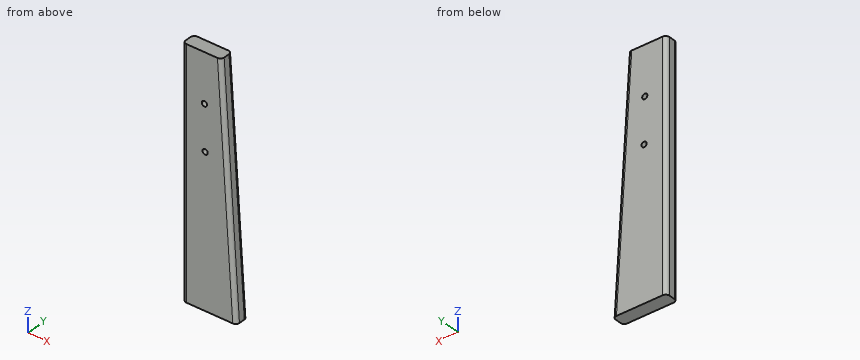
Autodesk Inventor part; units mm, degrees
ref_plane "YZ Plane" through (0, 0, 0) normal (1, 0, 0) x (0, 1, 0)
ref_plane "XZ Plane" through (0, 0, 0) normal (0, 1, 0) x (-1, 0, 0)
ref_plane "XY Plane" through (0, 0, 0) normal (0, 0, 1) x (1, 0, 0)
sketch "Skizze1" plane through (0, 0, 0) normal (0, 1, 0) x (-1, 0, 0)
  line L0 (0, 0) -> (10.3, 0)
  line L1 (10.3, 0) -> (10.3, -65)
  line L2 (10.3, -65) -> (-4.1, -65)
  line L3 (-4.1, -65) -> (0, 0)
  dimension "d0" = 65
  dimension "d1" = 14.4
  dimension "d2" = 10.3
extrude "Extrusion1" add sketch "Skizze1" along normal blind 3.6
sketch "Skizze2" plane through (0, 3.6, 0) normal (0, 1, 0) x (1, 0, 0)
  line L0 (-10.3, 65) -> (-10.3, 0)
  line L1 (-10.3, 0) -> (-10.3, 13)
  line L2 (-10.3, 0) -> (-10.3, 25)
  line L3 (-10.3, 13) -> (-4.5, 13)
  line L4 (-10.3, 25) -> (-4.3, 25)
  point P0 (0, 0)
  dimension "d5" = 13
  dimension "d6" = 25
  dimension "d7" = 5.8
  dimension "d8" = 6
hole "Bohrung1" at (-4.5, 3.6, -13) at (-4.3, 3.6, -25) direction (0, -1, 0) diameter 1.4 end through all
fillet "Rundung1" radius 1 4 edges at (-10.3, 3.6, -32.5) (-10.3, 0, -32.5) (2.05, 3.6, -32.5) (2.05, 0, -32.5)
properties part number "Brillenbuegel"
Source: CAD feature listing. Evaluate the final solid. Frame: model axes, mm. Give positions to 0.01 mm unless a question says otherwise; leave off trailing zeros. Order: outer loops, then holes, each group sorted by start corner. A loop starts at its lowest first (then second) coordinate and runs counter-clockwise, first axis right, second up. Notation, with made-up numbers: (74, 45.25) -> (128, 45.25) arc R30 ccw to (128, 78.25) -> close; hole circle Ø11 at (32, -34.75). An arc over 180 degrees is marked (long way). Write item = value, one per line.
Item 1: Section query A-A (y = 1.7). Output: boundary loops of the cut face in (x, z), then the cut area to 3 significant figures.
Check result:
outline = (-10.3, -65) -> (4.1, -65) -> (0, 0) -> (-10.3, 0) -> close; hole circle Ø1.4 at (-4.5, -13); hole circle Ø1.4 at (-4.3, -25)
area = 800 mm²
Item 2: Contact query for a flat-ended pin moving along its axis: pin 1 (1.5 mm diameter, centred on y = 0.5, z = -27, fed in from +X). Output: stop coordinate, or through.
Check result:
pin_1 = 1.74
Item 3: Ray query, probe 1 along Z at (x, y) = (-4.3, 2.4); probe 2 along X at (y, z) = (2.1, -13); probe 3 along X at (y, z) = (0.95, -25). Return the intervals inside material, ascending.
Check result:
probe_1 = -65 to -25.7, -24.3 to -13.67, -12.33 to 0
probe_2 = -10.3 to -5.2, -3.8 to 0.82
probe_3 = -10.3 to -5, -3.6 to 1.58
